```python
from build123d import *

# Parameters (mm, degrees)
BOSS_EXTRUDE1_DEPTH = 4
CUT_EXTRUDE1_DEPTH  = 1.5
SKETCH4_R           = 1.75
CUT_EXTRUDE3_DEPTH  = 17.5
SKETCH5_R           = 1.75
CUT_EXTRUDE4_DEPTH  = 17.5


with BuildPart() as part:
    # Sketch2 → Boss-Extrude1 (new body)
    with BuildSketch(Plane.XY):
        with BuildLine():
            Line((80, 37.5), (0, 37.5))
            ThreePointArc((0, 37.5), (-34.824248161, -13.911209149), (25.837194647, -27.178840534))
            ThreePointArc((25.837194647, -27.178840534), (35.524064233, -12.01211307), (37.029598104, 5.921052632))
            ThreePointArc((37.029598104, 5.921052632), (39.295298496, 13.988856845), (46.904157598, 17.5))
            Line((46.904157598, 17.5), (80, 17.5))
            ThreePointArc((80, 17.5), (90, 27.5), (80, 37.5))
        make_face()
    extrude(amount=BOSS_EXTRUDE1_DEPTH)

    # Sketch3 → Cut-Extrude1 (cut)
    with BuildSketch(Plane.XY.offset(4)):
        Polygon((26.483056848, -15.29), (26.483056848, -11.71), (23.382685902, -9.92), (20.282314957, -11.71), (20.282314957, -15.29), (23.382685902, -17.08), align=None)
        Polygon((0, 30.58), (-3.100370946, 28.79), (-3.100370946, 25.21), (0, 23.42), (3.100370946, 25.21), (3.100370946, 28.79), align=None)
        Polygon((-26.483056848, -15.29), (-23.382685902, -17.08), (-20.282314957, -15.29), (-20.282314957, -11.71), (-23.382685902, -9.92), (-26.483056848, -11.71), align=None)
    extrude(amount=-CUT_EXTRUDE1_DEPTH, mode=Mode.SUBTRACT)

    # Sketch4 → Cut-Extrude3 (cut)
    with BuildSketch(Plane.XY.offset(4)):
        with Locations((0, 27)):
            Circle(SKETCH4_R)
        with Locations((23.382685902, -13.5)):
            Circle(SKETCH4_R)
        with Locations((-23.382685902, -13.5)):
            Circle(SKETCH4_R)
    extrude(amount=-CUT_EXTRUDE3_DEPTH, mode=Mode.SUBTRACT)

    # Sketch5 → Cut-Extrude4 (cut)
    with BuildSketch(Plane.XY.offset(4)):
        with Locations((80, 27.5)):
            Circle(SKETCH5_R)
    extrude(amount=-CUT_EXTRUDE4_DEPTH, mode=Mode.SUBTRACT)


solid = part.part
```
Work out the finished part from the listing and answer in its coordinate system (mm). A direction names the side the tool comes from. Coordinates: 2 decimals unless noted, no trailing zeros. Write each loop counter-clockwise with the first axis right and the second up, starting at its lowest first coordinate (ties: lowest second). Pieces come first, ordered by that corner, then holes. Notation, with made-up numbers: (67.5, -5) - (85.5, -5) arc R13 ccw to (85.5, 19) - close; hole circle Ø11 at (-4.75, 26). An arc over 180 degrees is marked (long way). Answer as a JSON object with one key per item and string values.
Q1. Consider L1, parallel to X at y = -15, z = 2; L2, parallel to Y at x = 0, z = 1.8; L3, parallel to Y at x = 58, z = 0.25. Determine where each line is inside the solid, lowest interval first. Write a range as from..to.
Results list:
{"L1": "x = -34.37..-24.28, -22.48..22.48, 24.28..34.37", "L2": "y = -37.5..25.25, 28.75..37.5", "L3": "y = 17.5..37.5"}
Q2. Find section C-C (y = 20.5). Write down the section's boundary in (x, z), plus the area to 3 significant figures.
Results list:
{"outline": "(-31.4, 0) - (87.14, 0) - (87.14, 4) - (-31.4, 4) - close", "area": "474 mm^2"}
Q3. Given pin 1 Ø5.5 at (x, y) = (23.38, -13.5) entering from -Z; pin 2 Ø0.8 at (y, z) = (26.5, 3) entering from +X; pin 3 Ø1.2 at (y, z) = (-13.5, 3.5) entering from -X; pin 4 Ø1.6 at (y, z) = (26.5, 3) entering from -X, each flat-ended and moving along its own axis, determine where each tip first touches the part or whether it passes through.
Results list:
{"pin 1": "stops at z = 0", "pin 2": "stops at x = 89.98", "pin 3": "stops at x = -35.21", "pin 4": "stops at x = -27.31"}
Q4. For a pull along Y with two mould halves and no side action, classify faces 1 (the cylindrical face through (90, 27.3, 2)), 2 (the cylindrical face through (-0.228, 28.735, 1.268)), 3 (the flat face through (63, 17.5, 2)), 4 (the flat face through (-25, -15, 2.5)) as pulls with the +Y half, pulls with the -Y half, needs draft (parallel to the pull), parting line crosses it, or undercut.
Results list:
{"face 1": "parting line crosses it", "face 2": "undercut", "face 3": "pulls with the -Y half", "face 4": "undercut"}
Q5. Which of the six approach directions +Z, -Z, +X, -X, +Y, -Y give full straight-line access (tool end or side, diameter ignored) to faces 5 (the flat face through (22, -15, 2.5)), 6 (the cylindrical face through (25.05, -12.97, 1.27))?
Results list:
{"face 5": "+Z", "face 6": "+Z, -Z"}
Q6. Find section B-B (x = 55). Write down the section's boundary in (y, z).
Results list:
{"outline": "(17.5, 0) - (37.5, 0) - (37.5, 4) - (17.5, 4) - close"}
Q7. Find section A-A (z = 1.8). Write down the section's boundary in (x, y).
Results list:
{"outline": "(0, 37.5) arc R37.5 ccw (long way) to (37.03, 5.92) arc R10 cw to (46.9, 17.5) - (80, 17.5) arc R10 ccw to (80, 37.5) - close; hole circle Ø3.5 at (-23.38, -13.5); hole circle Ø3.5 at (0, 27); hole circle Ø3.5 at (23.38, -13.5); hole circle Ø3.5 at (80, 27.5)"}
